```python
from build123d import *

# Parameters (mm, degrees)
SKETCH1_W           = 132
SKETCH1_H           = 190
BOSS_EXTRUDE1_DEPTH = 7.5
SKETCH2_W           = 5
SKETCH2_H           = 7.5
BOSS_EXTRUDE2_DEPTH = 5
SKETCH3_R           = 2
CUT_EXTRUDE1_DEPTH  = 5
SKETCH4_R           = 3
CUT_EXTRUDE2_DEPTH  = 3.5


with BuildPart() as part:
    # Sketch1 → Boss-Extrude1 (new body)
    with BuildSketch(Plane.XY):
        Rectangle(SKETCH1_W, SKETCH1_H)
    extrude(amount=BOSS_EXTRUDE1_DEPTH)

    # Sketch2 → Boss-Extrude2 (add)
    with BuildSketch(Plane(origin=(0, -95, 0), x_dir=(-1, 0, 0), z_dir=(0, -1, 0))):
        with BuildLine():
            ThreePointArc((71, 0), (74.75, -3.75), (71, -7.5))
            Line((71, -7.5), (71, 0))
        make_face()
        with Locations((68.5, -3.75)):
            Rectangle(SKETCH2_W, SKETCH2_H)
        with BuildLine():
            ThreePointArc((-71, -7.5), (-74.75, -3.75), (-71, 0))
            Line((-71, 0), (-71, -7.5))
        make_face()
        with Locations((-68.5, -3.75)):
            Rectangle(SKETCH2_W, SKETCH2_H)
    extrude(amount=-BOSS_EXTRUDE2_DEPTH)

    # Sketch3 → Cut-Extrude1 (cut)
    with BuildSketch(Plane(origin=(0, -95, 0), x_dir=(-1, 0, 0), z_dir=(0, -1, 0))):
        with Locations((71, -3.75)):
            Circle(SKETCH3_R)
        with Locations((-71, -3.75)):
            Circle(SKETCH3_R)
    extrude(amount=-CUT_EXTRUDE1_DEPTH, mode=Mode.SUBTRACT)

    # Sketch4 → Cut-Extrude2 (cut)
    with BuildSketch(Plane(origin=(0, -95, 0), x_dir=(-1, 0, 0), z_dir=(0, -1, 0))):
        with Locations((71, -3.75)):
            Circle(SKETCH4_R)
        with Locations((-71, -3.75)):
            Circle(SKETCH4_R)
    extrude(amount=-CUT_EXTRUDE2_DEPTH, mode=Mode.SUBTRACT)


solid = part.part
```
Could you check a few things on this model? Use its own coordinates, in mm. A direction names the side the tool comes from. Coordinates: 2 decimals unless noted, no trailing zeros. Write each loop counter-clockwise with the first axis right and the second up, starting at its lowest first coordinate (ties: lowest second). Pieces come first, ordered by that corner, then holes. Notation, with made-up numbers: (40, -32) - (61, -32) arc R24 ccw to (61, -18) - close; hole circle Ø1 at (82, -35.75). An arc over 180 degrees is marked (long way). Use a Markdown table: item, result.
Q1. Imagine slicing it at A-A (z = 3.75). List the corners of the cut face in (x, y) for me.
Geometry check:
| item | result |
|---|---|
| outline | (-74.75, -95) - (-74, -95) - (-74, -91.5) - (-73, -91.5) - (-73, -90) - (-74.75, -90) - close; (-69, -91.5) - (-68, -91.5) - (-68, -95) - (68, -95) - (68, -91.5) - (69, -91.5) - (69, -90) - (66, -90) - (66, 95) - (-66, 95) - (-66, -90) - (-69, -90) - close; (73, -91.5) - (74, -91.5) - (74, -95) - (74.75, -95) - (74.75, -90) - (73, -90) - close |
Q2. Please list where these lines run through material, in increasing order: L1, parallel to X at y = -92.65, z = 3.75; L2, parallel to Z at x = -71, y = -92.55; L3, parallel to X at y = -19.5, z = 0.5.
Geometry check:
| item | result |
|---|---|
| L1 | x = -74.75 to -74, -68 to 68, 74 to 74.75 |
| L2 | z = 0 to 0.75, 6.75 to 7.5 |
| L3 | x = -66 to 66 |
Q3. I'm going to push flat-ended pins straight in: pin 1 Ø4 at (x, z) = (69.5, 3) entering from +Y; pin 2 Ø1 at (y, z) = (41.5, 6) entering from -X; pin 3 Ø1.8 at (x, z) = (-71, 4.5) entering from -Y; pin 4 Ø4 at (y, z) = (-16.5, 2) entering from +X. Where does each tip first touch, or does it pass through?
Geometry check:
| item | result |
|---|---|
| pin 1 | stops at y = -90 |
| pin 2 | stops at x = -66 |
| pin 3 | passes through |
| pin 4 | stops at x = 66 |
Q4. Which directions (+Z, -Z, +X, -X, +Y, -Y) give clear straight access to the entire face, cutting with the end or side of a thin tool? Please do faces 4 (the cylindrical face through (74.75, -92.54, 3.83)), 5 (the flat face through (66, 1, 4)), 6 (the flat face through (1, -1, 7.5)), 7 (the cylindrical face through (73.381, -93.274, 5.575)), 8 (the flat face through (-68, -90, 4)).
Geometry check:
| item | result |
|---|---|
| face 4 | +X, +Y, -Y |
| face 5 | +Z, -Z, +X, +Y |
| face 6 | +Z, +X, -X, +Y, -Y |
| face 7 | -Y |
| face 8 | +Z, -Z, -X, +Y |
Q5. Thinking about a two-plate mould opening in Z: for faces 1 (the cylindrical face through (-74.75, -92.54, 3.67)), 2 (the flat face through (-66, 1, 4)), 3 (the flat face through (70, -91.5, 6)), which applies, +Z half, -Z half, draft (parallel to the pull), parting line (faces both ways), or undercut?
Geometry check:
| item | result |
|---|---|
| face 1 | parting line |
| face 2 | draft |
| face 3 | undercut |
Q6. Imagine slicing it at B-B (y = 0). List the corners of the cut face in (x, z) for me.
Geometry check:
| item | result |
|---|---|
| outline | (-66, 0) - (66, 0) - (66, 7.5) - (-66, 7.5) - close |
